Build history of the part. All positions in model axes, mm. Coordinates: 2 decimals unless noted, no trailing zeros. Loops run counter-clockwise (first coordinate to the right, second up) from the corner with the lowest first, then second, coordinate; pieces in that order, holes last.
Item 1: Flat gauge pins, fed straight in: pin 1 (2 mm diameter, centred on x = 2, z = 5, fed in from -Y); pin 2 (2 mm diameter, centred on x = -4.5, z = 2.5, fed in from +Y). Where does each tip first touch, or does it go through?
Item 2: Cut at A-A (y = 0). List the corners of the cut face in (x, z), and give its area (3 significant figures).
Item 3: Cut at D-D (x = 4.25). List the corners of the cut face in (y, z), and give its area (3 significant figures).
Item 4: Mould opens along X. For faces 1 (the face through (-4.69, -5.208, 3.944)), 2 (the face through (-0.867, -3.905, 3.944)), 3 (the face through (-5, 0, 8)) say: released by +X, released by -X, zero draft, split by the parting line, or undercut.
Item 5: Drill centre lines: line 1 along Y through (x, z) = (0, 3); line 2 along Y through (x, z) = (-8.5, 2.5); line 3 along X through (y, z) = (1, 4.5). Where is each one in solid material? Low to high.
Item 6: Cut at B-B (x = -7). List the corners of the cut face in (y, z), and give its area (3 significant figures).
Item 7: Cut at C-C (z = 1.5). List the corners of the cut face in (x, y).
from build123d import *

# Parameters (mm, degrees)
F0_R     = 4
F1_DEPTH = 8


with BuildPart() as f1:
    # F0 (on Top) → F1 (new body)
    with BuildSketch(Plane.XY):
        with BuildLine():
            Line((-9.249722, -4.437107), (0, -6))
            ThreePointArc((0, -6), (6, 0), (0, 6))
            Line((0, 6), (-9.249722, 4.437107))
            ThreePointArc((-9.249722, 4.437107), (-10.32327, 4.114084), (-11.283653, 3.535714))
            ThreePointArc((-11.283653, 3.535714), (-11.450778, 2.13141), (-10.046474, 1.964286))
            ThreePointArc((-10.046474, 1.964286), (-6, 0), (-10.046474, -1.964286))
            ThreePointArc((-10.046474, -1.964286), (-11.450778, -2.13141), (-11.283653, -3.535714))
            ThreePointArc((-11.283653, -3.535714), (-10.32327, -4.114084), (-9.249722, -4.437107))
        make_face()
        Circle(F0_R, mode=Mode.SUBTRACT)
    extrude(amount=F1_DEPTH)


solid = f1.part
Filled sheet:
1. pin 1: stops at y = -5.92
1. pin 2: stops at y = 5.41
2. outline: (-6, 0) - (-4, 0) - (-4, 8) - (-6, 8) - close; (4, 0) - (6, 0) - (6, 8) - (4, 8) - close
2. area: 32.0 mm2
3. outline: (-4.24, 0) - (4.24, 0) - (4.24, 8) - (-4.24, 8) - close
3. area: 67.8 mm2
4. face 1: released by -X
4. face 2: undercut
4. face 3: zero draft
5. line 1: y = -6 to -4, 4 to 6
5. line 2: y = -4.56 to -2.5, 2.5 to 4.56
5. line 3: x = -6.21 to -3.87, 3.87 to 5.92
6. outline: (-4.82, 0) - (-2, 0) - (-2, 8) - (-4.82, 8) - close; (2, 0) - (4.82, 0) - (4.82, 8) - (2, 8) - close
6. area: 45.1 mm2
7. outline: (-11.28, -3.54) arc R4.5 ccw to (-9.25, -4.44) - (0, -6) arc R6 ccw to (0, 6) - (-9.25, 4.44) arc R4.5 ccw to (-11.28, 3.54) arc R1 ccw to (-10.05, 1.96) arc R2.5 cw (long way) to (-10.05, -1.96) arc R1 ccw to start; hole circle Ø8 at (0, 0)
